from build123d import *

# Parameters (mm, degrees)
SKETCH1_W           = 20
SKETCH1_H           = 3
BOSS_EXTRUDE1_DEPTH = 20
SKETCH3_W           = 20
SKETCH3_H           = 7.5
BOSS_EXTRUDE2_DEPTH = 20
SKETCH4_W           = 20
SKETCH4_H           = 7.5
BOSS_EXTRUDE3_DEPTH = 20
SKETCH2_W           = 11.3
SKETCH2_H           = 3
CUT_EXTRUDE1_DEPTH  = 20
SKETCH5_W           = 13.8
SKETCH5_H           = 0.9
CUT_EXTRUDE2_DEPTH  = 20
SKETCH6_W           = 10.5
SKETCH6_H           = 6.6
CUT_EXTRUDE3_DEPTH  = 17.5
SKETCH7_W           = 10.5
SKETCH7_H           = 6.6
CUT_EXTRUDE4_DEPTH  = 17.5
SKETCH8_W           = 3
SKETCH8_H           = 2
CUT_EXTRUDE5_DEPTH  = 20
SKETCH9_W           = 20
SKETCH9_H           = 13.4
BOSS_EXTRUDE4_DEPTH = 24
SKETCH10_R          = 3.1
CUT_EXTRUDE6_DEPTH  = 19
SKETCH11_R          = 1.45
CUT_EXTRUDE7_DEPTH  = 20
SKETCH12_W          = 10
SKETCH12_H          = 7
CUT_EXTRUDE8_DEPTH  = 20


with BuildPart() as part:
    # Sketch1 → Boss-Extrude1 (new body)
    with BuildSketch(Plane.XY):
        with Locations((0.456431535, 1.363070539)):
            Rectangle(SKETCH1_W, SKETCH1_H)
    extrude(amount=-BOSS_EXTRUDE1_DEPTH)

    # Sketch3 → Boss-Extrude2 (add)
    with BuildSketch(Plane.XY):
        with Locations((0.456431535, 6.613070539)):
            Rectangle(SKETCH3_W, SKETCH3_H)
    extrude(amount=-BOSS_EXTRUDE2_DEPTH)

    # Sketch4 → Boss-Extrude3 (add)
    with BuildSketch(Plane.XY):
        with Locations((0.456431535, -3.886929461)):
            Rectangle(SKETCH4_W, SKETCH4_H)
    extrude(amount=-BOSS_EXTRUDE3_DEPTH)

    # Sketch2 → Cut-Extrude1 (cut)
    with BuildSketch(Plane.XY):
        with Locations((0.456431535, 1.363070539)):
            Rectangle(SKETCH2_W, SKETCH2_H)
    extrude(amount=-CUT_EXTRUDE1_DEPTH, mode=Mode.SUBTRACT)

    # Sketch5 → Cut-Extrude2 (cut)
    with BuildSketch(Plane.XY):
        with Locations((0.456431535, -0.586929461)):
            Rectangle(SKETCH5_W, SKETCH5_H)
        with Locations((0.456431535, 3.313070539)):
            Rectangle(SKETCH5_W, SKETCH5_H)
    extrude(amount=-CUT_EXTRUDE2_DEPTH, mode=Mode.SUBTRACT)

    # Sketch6 → Cut-Extrude3 (cut)
    with BuildSketch(Plane.XY):
        with Locations((0.456431535, 7.063070539)):
            Rectangle(SKETCH6_W, SKETCH6_H)
    extrude(amount=-CUT_EXTRUDE3_DEPTH, mode=Mode.SUBTRACT)

    # Sketch7 → Cut-Extrude4 (cut)
    with BuildSketch(Plane.XY):
        with Locations((0.456431535, -4.336929461)):
            Rectangle(SKETCH7_W, SKETCH7_H)
    extrude(amount=-CUT_EXTRUDE4_DEPTH, mode=Mode.SUBTRACT)

    # Sketch8 → Cut-Extrude5 (cut)
    with BuildSketch(Plane.XY):
        with Locations((8.956431535, 9.363070539)):
            Rectangle(SKETCH8_W, SKETCH8_H)
        with Locations((-8.043568465, -6.636929461)):
            Rectangle(SKETCH8_W, SKETCH8_H)
    extrude(amount=-CUT_EXTRUDE5_DEPTH, mode=Mode.SUBTRACT)

    # Sketch9 → Boss-Extrude4 (add)
    with BuildSketch(Plane.ZY.offset(9.543568465)):
        with Locations((-10, 10.663070539)):
            Rectangle(SKETCH9_W, SKETCH9_H)
    extrude(amount=BOSS_EXTRUDE4_DEPTH)

    # Sketch10 → Cut-Extrude6 (cut)
    with BuildSketch(Plane.XY):
        with Locations((-26.543568465, 11.363070539)):
            Circle(SKETCH10_R)
    extrude(amount=-CUT_EXTRUDE6_DEPTH, mode=Mode.SUBTRACT)

    # Sketch11 → Cut-Extrude7 (cut)
    with BuildSketch(Plane.XY):
        with Locations((-26.543568465, 11.363070539)):
            Circle(SKETCH11_R)
    extrude(amount=-CUT_EXTRUDE7_DEPTH, mode=Mode.SUBTRACT)

    # Sketch12 → Cut-Extrude8 (cut)
    with BuildSketch(Plane.XY):
        with Locations((-14.543568465, 13.863070539)):
            Rectangle(SKETCH12_W, SKETCH12_H)
    extrude(amount=-CUT_EXTRUDE8_DEPTH, mode=Mode.SUBTRACT)


solid = part.part
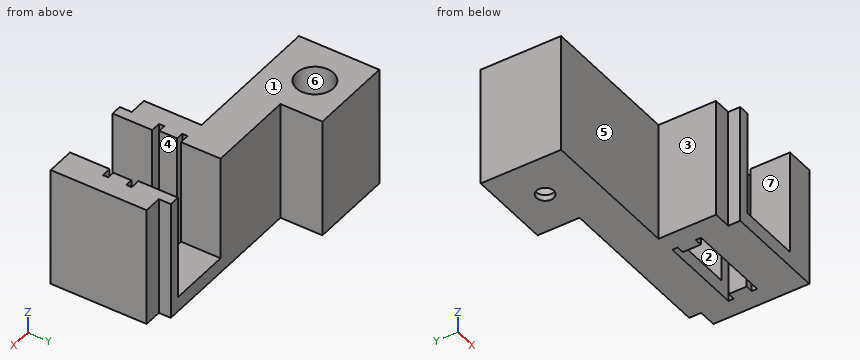
Could you check a few things on this model? Use its own coordinates, in mm. Face numbers are marked on the shaded views. A direction names the side the tool comes from. Round coordinates to 2 decimals unless told otherwise and drop trailing zeros. Loops run counter-clockwise (first coordinate to the right, second up) from the corner with the lowest first, then second, coordinate; pieces in that order, holes last. Notation, with made-up numbers: (52.25, -8) - (80.25, -8) arc R16 ccw to (80.25, 0) - close; hole circle Ø4 at (60, 57.25). An arc over 180 degrees is marked (long way). Write item = value, one per line.
1) Imagine slicing it at D-D (x = -24). Please give me the cut outline in (y, z).
Computed:
outline = (3.96, -20) - (17.36, -20) - (17.36, 0) - (13.14, 0) - (13.14, -19) - (9.59, -19) - (9.59, 0) - (3.96, 0) - close
2) If we mould it in two halves opening along X, with no side actions, what happens to the marked faces 1, 2 and 3? For each: pulls with the +X half, pulls with the -X half, needs draft (parallel to the pull), parting line crosses it, or undercut.
Computed:
face_1 = needs draft
face_2 = undercut
face_3 = pulls with the -X half
3) Imagine slicing it at B-B (z = -16.75). Give the number of separate pieces and of enclosed holes in the cut face, and give its area (3 significant figures).
Computed:
separate_pieces = 2
enclosed_holes = 1
area = 372 mm2
4) I'm going to push flat-ended pins straight in: P1, Ø5, axis at y = 0.5, z = -14.5, coming from the -X side; P2, Ø12, axis at x = 1.5, z = -16, coming from the +Y side; P3, Ø1.5, axis at x = 5, z = -17, coming from the -Y side; P4, Ø4, axis at x = -26.54, y = 11.36, coming from the +Z side. Where does each tip first touch, or does it pass through?
Computed:
P1 = -9.54
P2 = 10.36
P3 = -7.64
P4 = -19
5) Imagine slicing it at C-C (y = 7.5). Please give me the cut outline in (x, z).
Computed:
outline = (-33.54, -20) - (10.46, -20) - (10.46, 0) - (5.71, 0) - (5.71, -17.5) - (-4.79, -17.5) - (-4.79, 0) - (-33.54, 0) - close
6) On a 3-axis mill with a long thin cutter (end or side, diameter ignored), from which of +Z, -Z, +X, -X, +Y, -Y can I reach the whole of each face in a straight line? I mean the marked faces 4, 5, 6 and 7. Say none if no direction works.
Computed:
face_4 = +Z, -Z
face_5 = +Z, -Z, -X, -Y
face_6 = +Z
face_7 = +Z, +Y, -Y
7) I need wall thicknesses on line 1 along X through (y, z) = (2, -18.25); line 2 along X through (y, z) = (3.5, -18.75); line 3 along Y through (x, z) = (-22.5, -7.75). Which ranges of each line are inside material? Lowest first, please. Write a range as from..to.
Computed:
line_1 = -9.54..-5.19, 6.11..10.46
line_2 = -9.54..-6.44, 7.36..10.46
line_3 = 3.96..17.36
8) Imagine slicing it at A-A (x = -3.5). Please give me the cut outline in (y, z), and give its area (3 significant figures).
Computed:
outline = (-7.64, -20) - (-1.04, -20) - (-1.04, -17.5) - (-7.64, -17.5) - close; (3.76, -20) - (10.36, -20) - (10.36, -17.5) - (3.76, -17.5) - close
area = 33.0 mm2
